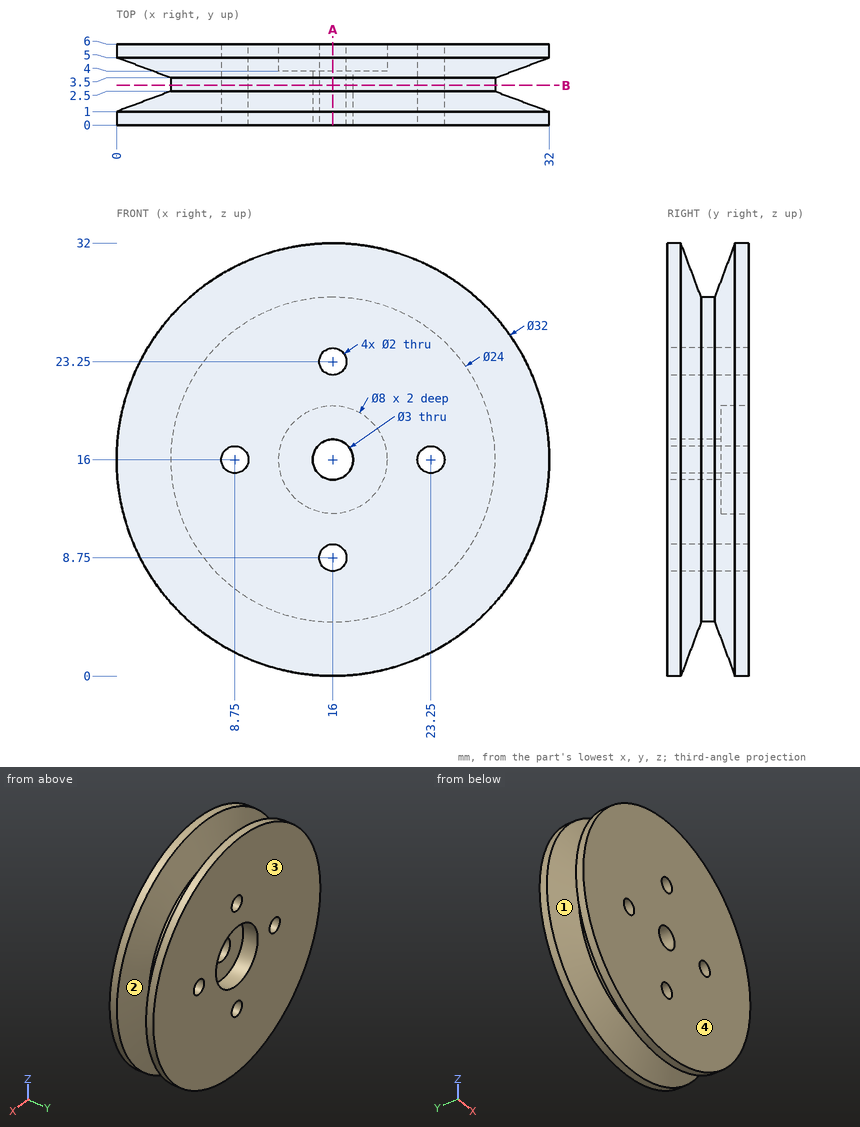
Answer from the drawing. Dimensions are ordinates in mm from the lowest x, y and z of the part. Round coordinates to 2 decimals unless told otherwise and drop trailing zeros. Write each loop counter-clockwise with the first axis right and the second up, starting at its lowest first coordinate (ties: lowest second). Pieces come first, ordered by that corner, then holes. Notation, with made-up numbers: (-14.5, -26.5) -> (-2.5, -26.5) arc R22 ccw to (-2.5, -11.5) -> close; hole circle Ø10 at (10.25, 31.5). An arc over 180 degrees is marked (long way). Write each question's results on one line, items separated by ' | '.
1) Flat-ended cylindrical pins translate along their axes: pin 1 (1.6 mm diameter, centred on x = 16, z = 8.75, fed in from -Y); pin 2 (6.5 mm diameter, centred on x = 16, z = 16, fed in from +Y); pin 3 (3 mm diameter, centred on y = 5, z = 26, fed in from -X). Find the tip coordinate at first contact, or state that the pin passes through.
Findings:
pin 1: passes through | pin 2: stops at y = 4 | pin 3: stops at x = 2.44
2) The part is cut by section B-B (y = 2.95). Write down the section's boundary in (x, z).
Findings:
outline: circle Ø24 at (16, 16); hole circle Ø2 at (8.75, 16); hole circle Ø3 at (16, 16); hole circle Ø2 at (16, 8.75); hole circle Ø2 at (16, 23.25); hole circle Ø2 at (23.25, 16)
3) For a pull along Y with two mould halves and no side action, classify the marked faces 1, 2, 3 and 4 as +Y half, -Y half, draft (parallel to the pull), parting line (faces both ways), or undercut.
Findings:
face 1: undercut | face 2: undercut | face 3: +Y half | face 4: -Y half
4) Consider line 1 along Z through (x, y) = (16, 5.6); line 2 along Y through (x, z) = (19.5, 16.5); line 3 along Y through (x, z) = (14.5, 29). Determine where each line is inside the solid, lowest interval first. Write a range as [from, to].
Findings:
line 1: z = [0, 7.75], [9.75, 12], [20, 22.25], [24.25, 32] | line 2: y = [0, 4] | line 3: y = [0, 2.09], [3.91, 6]
5) The part is cut by section A-A (x = 16). Write down the section's boundary in (y, z).
Findings:
outline: (0, 0) -> (1, 0) -> (2.5, 4) -> (3.5, 4) -> (5, 0) -> (6, 0) -> (6, 7.75) -> (0, 7.75) -> close; (0, 9.75) -> (6, 9.75) -> (6, 12) -> (4, 12) -> (4, 14.5) -> (0, 14.5) -> close; (0, 17.5) -> (4, 17.5) -> (4, 20) -> (6, 20) -> (6, 22.25) -> (0, 22.25) -> close; (0, 24.25) -> (6, 24.25) -> (6, 32) -> (5, 32) -> (3.5, 28) -> (2.5, 28) -> (1, 32) -> (0, 32) -> close
